For this review, take the finished solid that the model builds, in its own axes (mm). Coordinates: 2 decimals unless noted, no trailing zeros. Loops run counter-clockwise (first coordinate to the right, second up) from the corner with the lowest first, then second, coordinate; pieces in that order, holes last.
1. Take a section at B-B, the plane x = -190.5. State the section outline as (y, z) points.
2. Clearance check with a flat-ended pin moving along its axis: P1, Ø6, axis at x = -42.5, y = -177.5, coming from the -Z side. State where the tip first meets the part, or that it passes through.
3. To check wall thickness, follow probe 1 along Y at (x, z) = (-166, 4); probe 2 along X at (y, z) = (-429.5, 5.25); probe 3 along Y at (x, z) = (-349.5, 1). State the ranges of each line that lie inside material, in increasing order.
4. Take a section at A-A, the plane y = -177. State the section outline as (x, z) points.
```python
from build123d import *

# Parameters (mm, degrees)
F1_DEPTH = 6.35


with BuildPart() as f1:
    # F0 (on Top) → F1 (new body)
    with BuildSketch(Plane.XY):
        with BuildLine():
            Line((0, -107.95), (0, 0))
            Line((0, 0), (-365, 0))
            Line((-365, 0), (-365, -39.912774))
            ThreePointArc((-365, -39.912774), (-362.265006, -37.252341), (-358.575, -36.281802))
            Line((-358.575, -36.281802), (-346.075, -36.281802))
            Line((-346.075, -36.281802), (-346.075, -28.2))
            ThreePointArc((-346.075, -28.2), (-345.19632, -26.07868), (-343.075, -25.2))
            Line((-343.075, -25.2), (-33, -25.2))
            ThreePointArc((-33, -25.2), (-30.87868, -26.07868), (-30, -28.2))
            Line((-30, -28.2), (-30, -50.7))
            Line((-30, -50.7), (-13, -50.7))
            ThreePointArc((-13, -50.7), (-11.585786, -51.285786), (-11, -52.7))
            Line((-11, -52.7), (-11, -58.7))
            ThreePointArc((-11, -58.7), (-11.585786, -60.114214), (-13, -60.7))
            Line((-13, -60.7), (-30, -60.7))
            Line((-30, -60.7), (-30, -73.2))
            ThreePointArc((-30, -73.2), (-30.87868, -75.32132), (-33, -76.2))
            Line((-33, -76.2), (-44.45, -76.2))
            Line((-44.45, -76.2), (-44.45, -425.800476))
            ThreePointArc((-44.45, -425.800476), (-41.503539, -428.826711), (-44.50342, -431.8))
            Line((-44.50342, -431.8), (-339.9, -431.8))
            ThreePointArc((-339.9, -431.8), (-342.02132, -430.92132), (-342.9, -428.8))
            Line((-342.9, -428.8), (-342.9, -107.95))
            Line((-342.9, -107.95), (-342.9, -76.2))
            Line((-342.9, -76.2), (-343.075, -76.2))
            ThreePointArc((-343.075, -76.2), (-345.19632, -75.32132), (-346.075, -73.2))
            Line((-346.075, -73.2), (-346.075, -51.281802))
            Line((-346.075, -51.281802), (-358.575, -51.281802))
            ThreePointArc((-358.575, -51.281802), (-362.265006, -50.311262), (-365, -47.650829))
            Line((-365, -47.650829), (-365, -107.95))
            Line((-365, -107.95), (-365, -476.25))
            Line((-365, -476.25), (0, -476.25))
            Line((0, -476.25), (0, -107.95))
        make_face()
    extrude(amount=F1_DEPTH)


solid = f1.part
```
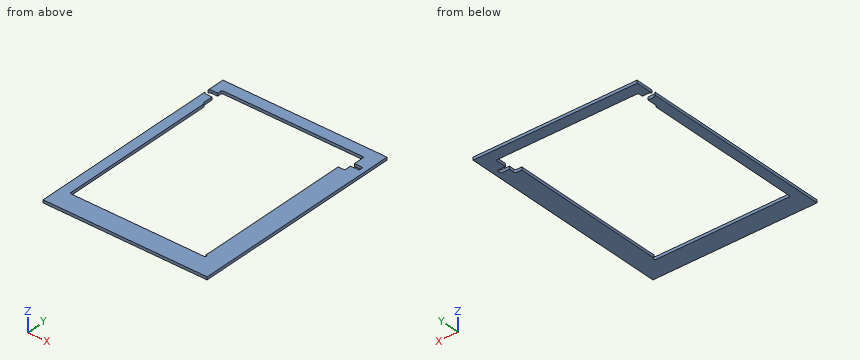
Results list:
1. outline: (-476.25, 0) - (-431.8, 0) - (-431.8, 6.35) - (-476.25, 6.35) - close; (-25.2, 0) - (0, 0) - (0, 6.35) - (-25.2, 6.35) - close
2. P1: stops at z = 0
3. probe 1: y = -476.25 to -431.8, -25.2 to 0
3. probe 2: x = -365 to -342.82, -41.59 to 0
3. probe 3: y = -476.25 to -51.28, -36.28 to 0
4. outline: (-365, 0) - (-342.9, 0) - (-342.9, 6.35) - (-365, 6.35) - close; (-44.45, 0) - (0, 0) - (0, 6.35) - (-44.45, 6.35) - close
